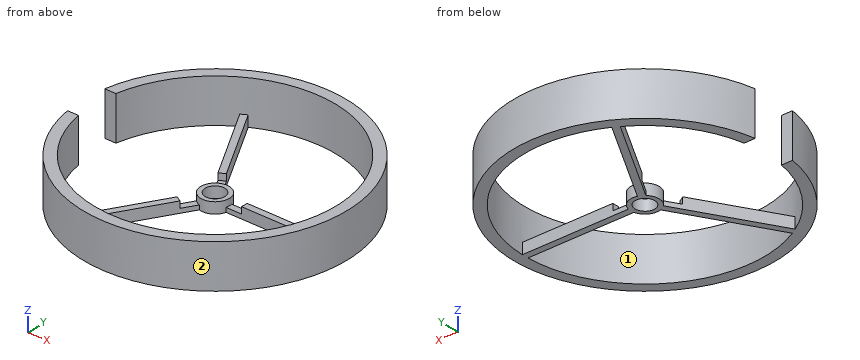
Autodesk Inventor part; units mm, degrees
ref_plane "YZ Plane" through (0, 0, 0) normal (1, 0, 0) x (0, 1, 0)
ref_plane "XZ Plane" through (0, 0, 0) normal (0, 1, 0) x (-1, 0, 0)
ref_plane "XY Plane" through (0, 0, 0) normal (0, 0, 1) x (1, 0, 0)
sketch "Sketch1" plane through (0, 0, 0) normal (0, 0, 1) x (1, 0, 0)
  circle A0 centre (0, 0) radius 60 construction
  line L0 (-59.1608, 10) -> (-59.1608, -10) construction
  circle A1 centre (0, 0) radius 55 construction
  line L1 (-59.1608, 10) -> (-54.0833, 10)
  line L2 (-59.1608, -10) -> (-54.0833, -10)
  arc A2 (-59.1608, -10) -> (-59.1608, 10) centre (0, 0) ccw
  arc A3 (-54.0833, -10) -> (-54.0833, 10) centre (0, 0) ccw
  circle A4 centre (0, 0) radius 4.5
  circle A5 centre (0, 0) radius 6.5
  line L3 (4.2426, 1.5) -> (59.9812, 1.5)
  line L4 (4.2426, -1.5) -> (59.9812, -1.5)
  arc A6 (4.2426, -1.5) -> (4.2426, 1.5) centre (0, 0) ccw
  arc A7 (59.9812, -1.5) -> (59.9812, 1.5) centre (0, 0) ccw
  line L5 (-3.4204, 2.9242) -> (-31.2897, 51.1953)
  line L6 (-0.8223, 4.4242) -> (-28.6916, 52.6953)
  line L7 (-0.8223, -4.4242) -> (-28.6916, -52.6953)
  line L8 (-3.4204, -2.9242) -> (-31.2897, -51.1953)
  arc A8 (-0.8223, 4.4242) -> (-3.4204, 2.9242) centre (0, 0) ccw
  arc A9 (-3.4204, -2.9242) -> (-0.8223, -4.4242) centre (0, 0) ccw
  arc A10 (-28.6916, 52.6953) -> (-31.2897, 51.1953) centre (0, 0) ccw
  arc A11 (-31.2897, -51.1953) -> (-28.6916, -52.6953) centre (0, 0) ccw
  point P0 (-59.1608, 0)
  dimension "d0" = 120
  dimension "d1" = 20
  dimension "d2" = 5
  dimension "d5" = 9
  dimension "d7" = 3
  dimension "d10" = 360
  dimension "d17" = 13
extrude "Extrusion1" add sketch "Sketch1" along normal blind 20 contours A2 L5 A3 L1 | A2 L6 A3 L5 | A2 L3 A3 L6 | L5 A4 L8 A5 | A5 L6 A4 L5 | A2 L4 A3 L3 | A5 L3 A4 L6 | L8 A4 L7 A5 | A2 L7 A3 L4 | A5 L4 A4 L3 | L7 A4 L4 A5 | L8 A2 L2 A3 | A3 L7 A2 L8
extrude "Extrusion2" add sketch "Sketch1" along normal blind 5 contours A2 L6 A3 L5 | A3 L6 A5 L5 | A5 L6 A4 L5 | A2 L4 A3 L3 | A3 L4 A5 L3 | L8 A4 L7 A5 | A5 L7 A3 L8 | A5 L4 A4 L3 | A3 L7 A2 L8
sketch "Sketch3" plane through (0, 0, 20) normal (0, 0, 1) x (1, 0, 0)
  circle A0 centre (0, 0) radius 4.5
  circle A1 centre (0, 0) radius 6.5
  point P0 (0, 0)
extrude "Extrusion3" cut sketch "Sketch3" against normal blind 15
sketch "Sketch4" plane through (0, 0, 5) normal (0, 0, 1) x (1, 0, 0)
  arc A0 (6.3246, 1.5) -> (-1.8632, 6.2272) centre (0, 0) ccw
  line L0 (54.9795, 1.5) -> (6.3246, 1.5)
  circle A1 centre (0, 0) radius 6.5
  circle A2 centre (0, 0) radius 13.5
  point P0 (0, 0)
  dimension "d18" = 27
extrude "Extrusion4" cut sketch "Sketch4" against normal blind 3
properties part number "AA051" material "ABS Plastic"
Input: part model. Units: mm. Frame: model coordinates. Face numbers are marked on the shaded views. Round coordinates to 2 decimals unless told otherwise and drop trailing zeros. Write each loop counter-clockwise with the first axis right and the second up, starting at its lowest first coordinate (ties: lowest second). Pieces come first, ordered by that corner, then holes.
1) Cut plane C-C (x = 26). Return the cut outline in (y, z).
2) Contact query for flat-ended pins moving along their axis: P1, Ø1, axis at x = -23.5, z = 3.5, coming from the +Y side; P2, Ø10, axis at x = -30, z = 10, coming from the +Y side; P3, Ø5, axis at x = -6, y = -8.5, coming from the +Z side; P4, Ø7, axis at x = 0, y = 0, coming from the -Z side. Output: stop coordinate, or through.
3) Ray query, L1, parallel to Y at x = 0, z = 2.3; L2, parallel to Y at x = 0, z = 15.25; L3, parallel to Y at x = 4, z = 2.5. Return the intervals inside material, ascending.
4) Cut plane B-B (y = 0). Return the cut outline in (x, z).
5) Cut plane A-A (x = 0). Return the cut outline in (y, z).
6) Draft query along X for the marked faces 1 and 2. Return one class per face: pulls with the +X half, pulls with the -X half, needs draft (parallel to the pull), parting line crosses it, or undercut.
7) Cut plane D-D (y = 20). Return the cut outline in (x, z), then the cut area to 3 significant figures.
Geometry says:
1. outline: (-54.07, 0) - (-48.47, 0) - (-48.47, 20) - (-54.07, 20) - close; (-1.5, 0) - (1.5, 0) - (1.5, 5) - (-1.5, 5) - close; (48.47, 0) - (54.07, 0) - (54.07, 20) - (48.47, 20) - close
2. P1: stops at y = 55.42
2. P2: stops at y = 54.54
2. P3: stops at z = 2
2. P4: passes through
3. L1: y = -60 to -55, -6.5 to -4.5, 4.5 to 6.5, 55 to 60
3. L2: y = -60 to -55, 55 to 60
3. L3: y = -59.87 to -54.85, -5.12 to -2.06, 2.06 to 5.12, 54.85 to 59.87
4. outline: (-6.5, 0) - (-4.5, 0) - (-4.5, 5) - (-6.5, 5) - close; (4.5, 0) - (60, 0) - (60, 20) - (55, 20) - (55, 5) - (13.5, 5) - (13.5, 2) - (6.5, 2) - (6.5, 5) - (4.5, 5) - close
5. outline: (-60, 0) - (-55, 0) - (-55, 20) - (-60, 20) - close; (-6.5, 0) - (-4.5, 0) - (-4.5, 5) - (-6.5, 5) - close; (4.5, 0) - (6.5, 0) - (6.5, 5) - (4.5, 5) - close; (55, 0) - (60, 0) - (60, 20) - (55, 20) - close
6. face 1: undercut
6. face 2: parting line crosses it
7. outline: (-56.57, 0) - (-51.23, 0) - (-51.23, 20) - (-56.57, 20) - close; (-13.28, 0) - (-9.81, 0) - (-9.81, 5) - (-13.28, 5) - close; (51.23, 0) - (56.57, 0) - (56.57, 20) - (51.23, 20) - close
7. area: 231 mm2
